The listing builds one solid part. Answer for the finished solid, in the listing's coordinates (mm). Give positions to 0.01 mm unless a question says otherwise; leave off trailing zeros. Loops run counter-clockwise (first coordinate to the right, second up) from the corner with the lowest first, then second, coordinate; pieces in that order, holes last.
Item 1: Each of these flat-tipped pins is pushed along its axis until it touches: pin 1 Ø3 at (x, y) = (0, 0) entering from +Z; pin 2 Ø1.5 at (x, z) = (-2, -1.5) entering from +Y. Where does it stop, or does it pass through?
Item 2: Consider line 1 along X through (y, z) = (-1, -1.45); line 2 along Y through (x, z) = (2.75, -1.75); line 3 along X through (y, z) = (-0.75, -0.6). Determine where each line is inside the solid, lowest interval first.
Item 3: Section A-A, the plane z = -1.4 is taken. Give the vertices of the cut face in (x, y), and give its area (3 significant figures).
from build123d import *

# Parameters (mm, degrees)
BASENUT_START = -2.8956
BASENUTSKE_R  = 1.35255
BASENUT_DEPTH = 2.8956


with BuildPart() as part:
    # BaseNutSke → BaseNut (new body)
    with BuildSketch(Plane.XY.offset(BASENUT_START)):
        Polygon((3.9624, 2.287692707), (3.9624, -2.287692707), (0, -4.575385413), (-3.9624, -2.287692707), (-3.9624, 2.287692707), (0, 4.575385413), align=None)
        Circle(BASENUTSKE_R, mode=Mode.SUBTRACT)
    extrude(amount=BASENUT_DEPTH)

    # Sketch4 → Single-Chamfer (revolve, cut)
    with BuildSketch(Plane(origin=(0, 0, 0), x_dir=(0, 0, -1), z_dir=(1, 0, 0))):
        Polygon((0, 3.9624), (-12.7, 3.9624), (-12.7, 17.275385413), (0.353907293, 17.275385413), (0.353907293, 4.575385413), align=None)
    revolve(axis=Axis((0, 0, 0), (0, 0, -1)), mode=Mode.SUBTRACT)

    # EndChamferSketch → EndChamfer (revolve, cut)
    with BuildSketch(Plane(origin=(0, 0, 0), x_dir=(0, 0, -1), z_dir=(1, 0, 0)), mode=Mode.PRIVATE) as endchamfer_sk:
        Polygon((2.8702, 1.7526), (2.562070172, 1.312545), (2.921, 1.312545), (2.921, 1.7526), align=None)
        Polygon((-0.0508, 1.7526), (0, 1.7526), (0.308129828, 1.312545), (-0.0508, 1.312545), align=None)
    revolve(endchamfer_sk.sketch.rotate(Axis((0, 0, -25.037505729), (0, 0, -1)), 90), axis=Axis((0, 0, -25.037505729), (0, 0, -1)), mode=Mode.SUBTRACT)


solid = part.part
Worked answers:
1. pin 1: stops at z = -0.18
1. pin 2: stops at y = 3.85
2. line 1: x = -3.96 to -0.91, 0.91 to 3.96
2. line 2: y = -2.99 to 2.99
2. line 3: x = -3.96 to -1.13, 1.13 to 3.96
3. outline: (-3.96, -2.29) - (0, -4.58) - (3.96, -2.29) - (3.96, 2.29) - (0, 4.58) - (-3.96, 2.29) - close; hole circle Ø2.71 at (0, 0)
3. area: 48.6 mm2
